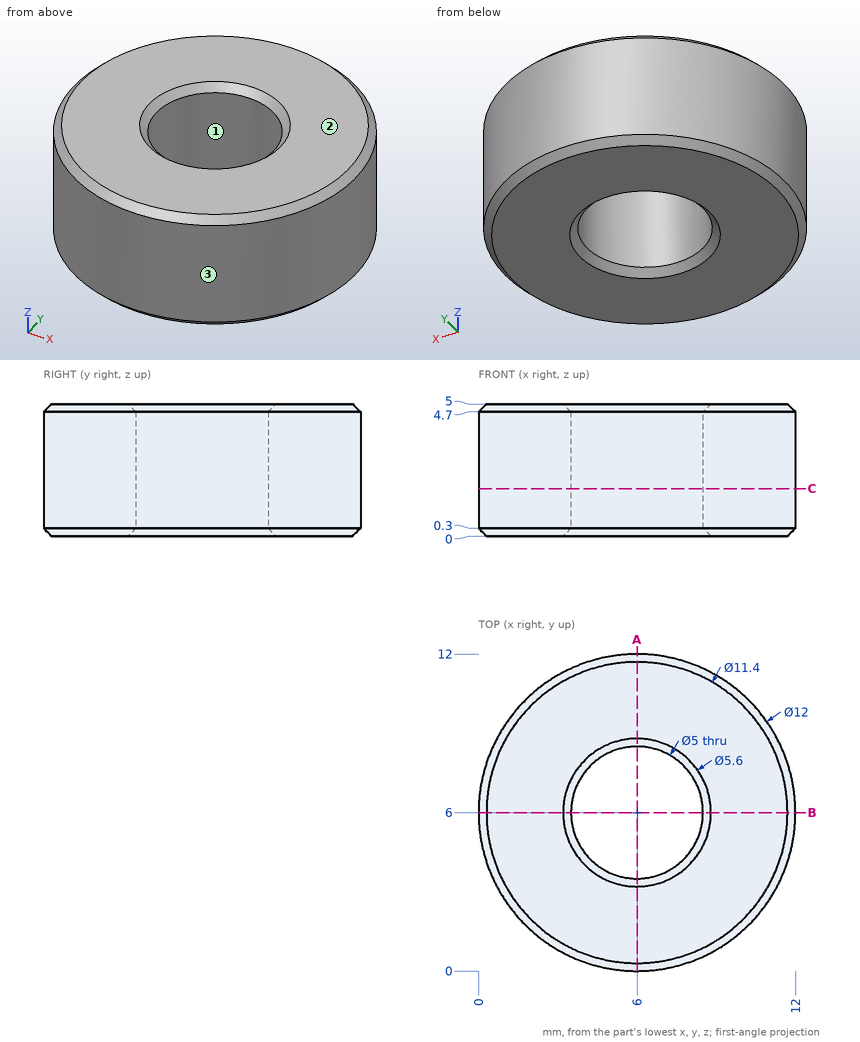
Check sheet for the drawn part. Datum: minimum x, y, z corner. Units: mm. Give positions to 0.01 mm unless a question says otherwise; leave off trailing zeros. Order: outer loops, then holes, each group sorted by start corner. A loop starts at its lowest first (then second) coordinate and runs counter-clockwise, first axis right, second up. Notation, with made-up numbers: (44.5, 24) - (73.5, 24) arc R28 ccw to (73.5, 60) - close; hole circle Ø5 at (-7, 64). An arc over 180 degrees is marked (long way). Answer as a JSON object with one key per item and string values.
(1) Depth check by flat-ended pin: pin 1 Ø3 at (x, y) = (6, 6) entering from -Z; pin 2 Ø6 at (x, y) = (3, 5.5) entering from -Z; pin 3 Ø3 at (y, z) = (9, 3.5) entering from -X; pin 4 Ø1 at (y, z) = (10.5, 2.5) entering from -X. Enter the tip coordinate at first touch or a pass-through.
Report:
{"pin 1": "through", "pin 2": "z = 0", "pin 3": "x = 0.19", "pin 4": "x = 1.53"}
(2) Cross-section at A-A (x = 6). Record the cut outline in (y, z), then the cut area to 3 significant figures.
Report:
{"outline": "(0, 0.3) - (0.3, 0) - (3.2, 0) - (3.5, 0.3) - (3.5, 4.7) - (3.2, 5) - (0.3, 5) - (0, 4.7) - close; (8.5, 0.3) - (8.8, 0) - (11.7, 0) - (12, 0.3) - (12, 4.7) - (11.7, 5) - (8.8, 5) - (8.5, 4.7) - close", "area": "34.6 mm^2"}
(3) Draft check along X on the marked faces 1, 2 and 3. Enter one of: released by +X, released by -X, zero draft, split by the parting line, or undercut.
Report:
{"face 1": "undercut", "face 2": "zero draft", "face 3": "split by the parting line"}
(4) Material ranges on line 1 (Y direction, x = 6, z = 2.95); line 2 (Y direction, x = 6.5, z = 3.35); line 3 (X direction, y = 7.5, z = 4.3), recorded low to high.
Report:
{"line 1": "0 to 3.5, 8.5 to 12", "line 2": "0.02 to 3.55, 8.45 to 11.98", "line 3": "0.19 to 4, 8 to 11.81"}
(5) Cross-section at C-C (z = 1.8). Record the cut outline in (x, y).
Report:
{"outline": "circle Ø12 at (6, 6); hole circle Ø5 at (6, 6)"}
